Geometry check sheet. Reference: the model listing, model coordinates, mm. A direction names the side the tool comes from. Coordinates: 2 decimals unless noted, no trailing zeros. Loops run counter-clockwise (first coordinate to the right, second up) from the corner with the lowest first, then second, coordinate; pieces in that order, holes last. Notation, with made-up numbers: (7.5, -25) - (65.5, -25) arc R21 cw to (65.5, 0) - close; hole circle Ø5 at (4.5, 52). An arc over 180 degrees is marked (long way). One line per item, written item: value.
from build123d import *

# Parameters (mm, degrees)
SKETCH1_W           = 42
SKETCH1_H           = 42
BOSS_EXTRUDE1_DEPTH = 40
SKETCH2_R           = 11
BOSS_EXTRUDE2_DEPTH = 2
SKETCH3_R           = 2.5
BOSS_EXTRUDE3_DEPTH = 24
CHAMFER1_SIZE       = 3
SKETCH4_R           = 1.5
CUT_EXTRUDE1_DEPTH  = 10


with BuildPart() as part:
    # Sketch1 → Boss-Extrude1 (new body)
    with BuildSketch(Plane.XY):
        Rectangle(SKETCH1_W, SKETCH1_H)
    extrude(amount=BOSS_EXTRUDE1_DEPTH)

    # Sketch2 → Boss-Extrude2 (add)
    with BuildSketch(Plane.XY.offset(40)):
        Circle(SKETCH2_R)
    extrude(amount=BOSS_EXTRUDE2_DEPTH)

    # Sketch3 → Boss-Extrude3 (add)
    with BuildSketch(Plane.XY.offset(42)):
        Circle(SKETCH3_R)
    extrude(amount=BOSS_EXTRUDE3_DEPTH)

    # Chamfer1
    chamfer1_edges = [part.edges().sort_by_distance(p)[0] for p in [
        (21, -21, 20),
        (-21, -21, 20),
        (-21, 21, 20),
        (21, 21, 20),
    ]]
    chamfer(chamfer1_edges, length=CHAMFER1_SIZE)

    # Sketch4 → Cut-Extrude1 (cut)
    with BuildSketch(Plane.XY.offset(40)):
        with Locations((-15.75, 15.75)):
            Circle(SKETCH4_R)
        with Locations((15.75, 15.75)):
            Circle(SKETCH4_R)
        with Locations((-15.75, -15.75)):
            Circle(SKETCH4_R)
        with Locations((15.75, -15.75)):
            Circle(SKETCH4_R)
    extrude(amount=-CUT_EXTRUDE1_DEPTH, mode=Mode.SUBTRACT)


solid = part.part
(1) Cross-section at D-D on y = 8. Record the cut outline in (x, z).
Reply:
outline: (-21, 0) - (21, 0) - (21, 40) - (7.55, 40) - (7.55, 42) - (-7.55, 42) - (-7.55, 40) - (-21, 40) - close
(2) Release check for a two-part mould opening along X. For faces 3 (the face through (0, 21, 20)), 4 (the face through (-16, 16, 30)), 5 (the face through (-21, 0, 20)), 6 (the face through (-2.38, -10.74, 40.99)) record: pulls with the +X half, pulls with the -X half, needs draft (parallel to the pull), parting line crosses it, or undercut.
Reply:
face 3: needs draft
face 4: undercut
face 5: pulls with the -X half
face 6: parting line crosses it
(3) Cross-section at A-A on x = 0. Record the cut outline in (y, z).
Reply:
outline: (-21, 0) - (21, 0) - (21, 40) - (11, 40) - (11, 42) - (2.5, 42) - (2.5, 66) - (-2.5, 66) - (-2.5, 42) - (-11, 42) - (-11, 40) - (-21, 40) - close
(4) Cross-section at C-C on z = 45. Record the cut outline in (x, y), and give its area (3 significant figures).
Reply:
outline: circle Ø5 at (0, 0)
area: 19.6 mm2
(5) Go/stop test with flat-tipped pins: pin 1 Ø0.9 at (x, y) = (-16, -16) entering from +Z; pin 2 Ø5 at (x, z) = (6, 50.5) entering from +Y; pin 3 Ø12 at (x, y) = (-14.5, -7.5) entering from +Z; pin 4 Ø3.5 at (x, y) = (15.75, 15.75) entering from +Z. Record where each tip stops, or that it passes through.
Reply:
pin 1: z = 30
pin 2: through
pin 3: z = 42
pin 4: z = 40
(6) Access from +Z, -Z, +X, -X, +Y, -Y to the whole of each face (thin tool, end or side, straight path). Record for faces 1 (the face through (-17.25, -15.68, 35.07)), 2 (the face through (20, 19, 20)).
Reply:
face 1: +Z
face 2: +Z, -Z, +X, +Y
(7) Material ranges on probe 1 along X at (y, z) = (-15, 36); probe 2 along Z at (x, y) = (4.5, -4); probe 3 along Z at (x, y) = (-10.5, 16), recorded low to high. Write a range as from..to.
Reply:
probe 1: -21..-17.05, -14.45..14.45, 17.05..21
probe 2: 0..42
probe 3: 0..40
